from build123d import *

# Parameters (mm, degrees)
BOSS_EXTRUDE1_DEPTH     = 20.95
BOSS_EXTRUDE2_DEPTH     = 9.05
SKETCH6_R               = 2
CUT_EXTRUDE2_DEPTH      = 10
CUT_EXTRUDE3_DEPTH      = 2.75
SKETCH8_W               = 8.290514233
SKETCH8_H               = 3.25
CUT_EXTRUDE4_DEPTH      = 1
CUT_EXTRUDE4_DEPTH_BACK = 31
SKETCH11_R              = 11.15
BEARING_HOLE_DEPTH      = 7.3
SKETCH9_W               = 12.1
SKETCH9_H               = 21.5
WIRE_HOLE_DEPTH         = 15.75
SKETCH12_W              = 46
SKETCH12_H              = 30
BOSS_EXTRUDE3_DEPTH     = 0.0001
BOSS_EXTRUDE4_DEPTH     = 7.5
BOSS_EXTRUDE5_DEPTH     = 7.5
BOSS_EXTRUDE9_DEPTH     = 2.5
SKETCH15_R              = 4
CUT_EXTRUDE5_DEPTH      = 49.5
SKETCH17_R              = 6.169612062
BOSS_EXTRUDE6_DEPTH     = 10
SKETCH18_R              = 3.85
BOSS_EXTRUDE7_DEPTH     = 14
SKETCH19_R              = 4.675
CUT_EXTRUDE6_DEPTH      = 2
SKETCH24_R              = 3.5
CUT_EXTRUDE7_DEPTH      = 23.7
FILLET1_R               = 0.5
SKETCH25_W              = 8.843315878
SKETCH25_H              = 4.834346013
BOSS_EXTRUDE10_DEPTH    = 2
SKETCH27_W              = 12.1
SKETCH27_H              = 21.5
CUT_EXTRUDE8_DEPTH      = 50.7501
BOSS_EXTRUDE11_DEPTH    = 14.7501
SKETCH29_W              = 15.1
SKETCH29_H              = 3
CUT_EXTRUDE9_DEPTH      = 20.95
SKETCH30_R              = 4
CUT_EXTRUDE10_DEPTH     = 14
CUT_EXTRUDE11_DEPTH     = 3


with BuildPart() as part:
    # Sketch2 → Boss-Extrude1 (new body)
    with BuildSketch(Plane.XY):
        with BuildLine():
            Line((-14.709485767, 40), (-23, 40))
            Line((-23, 40), (-23, 0))
            Line((-23, 0), (23, 0))
            Line((23, 0), (23, 40))
            Line((23, 40), (14.709485767, 40))
            ThreePointArc((14.709485767, 40), (0, 54.709485767), (-14.709485767, 40))
        make_face()
        with BuildLine():
            Line((-7.55, 18.241114036), (-7.55, 14.75))
            Line((-7.55, 14.75), (7.55, 14.75))
            Line((7.55, 14.75), (7.55, 18.241114036))
            Line((7.55, 18.241114036), (9.25, 18.241114036))
            Line((9.25, 18.241114036), (9.25, 21.160258306))
            ThreePointArc((9.25, 21.160258306), (0, 46.25), (-9.25, 21.160258306))
            Line((-9.25, 21.160258306), (-9.25, 18.241114036))
            Line((-9.25, 18.241114036), (-7.55, 18.241114036))
        make_face(mode=Mode.SUBTRACT)
    extrude(amount=BOSS_EXTRUDE1_DEPTH)

    # Sketch3 → Boss-Extrude2 (add)
    with BuildSketch(Plane.XY):
        with BuildLine():
            Line((-14.709485767, 40), (-23, 40))
            Line((-23, 40), (-23, 0))
            Line((-23, 0), (23, 0))
            Line((23, 0), (23, 40))
            Line((23, 40), (14.709485767, 40))
            ThreePointArc((14.709485767, 40), (0, 54.709485767), (-14.709485767, 40))
        make_face()
    extrude(amount=-BOSS_EXTRUDE2_DEPTH)

    # Sketch6 → Cut-Extrude2 (cut)
    with BuildSketch(Plane.XY.offset(20.95)):
        with Locations((-17.5, 32)):
            Circle(SKETCH6_R)
        with Locations((17.5, 32)):
            Circle(SKETCH6_R)
    extrude(amount=-CUT_EXTRUDE2_DEPTH, mode=Mode.SUBTRACT)

    # Sketch7 → Cut-Extrude3 (cut)
    with BuildSketch(Plane.XY.offset(20.95)):
        with BuildLine():
            Line((-17.5, 35.75), (17.5, 35.75))
            ThreePointArc((17.5, 35.75), (21.25, 32), (17.5, 28.25))
            Line((17.5, 28.25), (-17.5, 28.25))
            ThreePointArc((-17.5, 28.25), (-21.25, 32), (-17.5, 35.75))
        make_face()
    extrude(amount=-CUT_EXTRUDE3_DEPTH, mode=Mode.SUBTRACT)

    # Sketch8 → Cut-Extrude4 (cut, two sides)
    with BuildSketch(Plane.XY.offset(20.95)) as cut_extrude4_sk:
        with Locations((-18.854742884, 38.375)):
            Rectangle(SKETCH8_W, SKETCH8_H)
        with Locations((18.854742884, 38.375)):
            Rectangle(SKETCH8_W, SKETCH8_H)
    extrude(amount=CUT_EXTRUDE4_DEPTH, mode=Mode.SUBTRACT)
    extrude(cut_extrude4_sk.sketch, amount=-CUT_EXTRUDE4_DEPTH_BACK, mode=Mode.SUBTRACT)

    # Sketch11 → Bearing Hole (cut)
    with BuildSketch(Plane(origin=(0, 0, -9.05), x_dir=(-1, 0, 0), z_dir=(0, 0, -1))):
        with Locations((0, 40)):
            Circle(SKETCH11_R)
    extrude(amount=-BEARING_HOLE_DEPTH, mode=Mode.SUBTRACT)

    # Sketch9 → Wire Hole (cut, through all)
    with BuildSketch(Plane(origin=(0, 14.75, -19.25), x_dir=(-1, 0, 0), z_dir=(0, 1, 0))):
        with Locations((0, 26.95)):
            Rectangle(SKETCH9_W, SKETCH9_H)
    extrude(amount=-WIRE_HOLE_DEPTH, mode=Mode.SUBTRACT)

    # Sketch12 → Boss-Extrude3 (add)
    with BuildSketch(Plane.XZ):
        with Locations((0, 5.95)):
            Rectangle(SKETCH12_W, SKETCH12_H)
    extrude(amount=BOSS_EXTRUDE3_DEPTH)

    # Sketch13 → Boss-Extrude4 (add)
    with BuildSketch(Plane(origin=(23, 0, 0), x_dir=(0, 0, -1), z_dir=(1, 0, 0))):
        with BuildLine():
            Line((-20.95, -0.0001), (-20.95, -20.0001))
            ThreePointArc((-20.95, -20.0001), (-5.95, -35.0001), (9.05, -20.0001))
            Line((9.05, -20.0001), (9.05, -0.0001))
            Line((9.05, -0.0001), (-20.95, -0.0001))
        make_face()
    extrude(amount=-BOSS_EXTRUDE4_DEPTH)

    # Sketch14 → Boss-Extrude5 (add)
    with BuildSketch(Plane.ZY.offset(23)):
        with BuildLine():
            Line((-9.05, -20.0001), (-9.05, -0.0001))
            Line((-9.05, -0.0001), (20.95, -0.0001))
            Line((20.95, -0.0001), (20.95, -20.0001))
            ThreePointArc((20.95, -20.0001), (5.95, -35.0001), (-9.05, -20.0001))
        make_face()
    extrude(amount=-BOSS_EXTRUDE5_DEPTH)

    # Sketch21 → Boss-Extrude9 (add)
    with BuildSketch(Plane(origin=(23, 0, 0), x_dir=(0, 0, -1), z_dir=(1, 0, 0))):
        with BuildLine():
            Line((-20.95, -20.0001), (-20.95, 36.75))
            Line((-20.95, 36.75), (9.05, 36.75))
            Line((9.05, 36.75), (9.05, -20.0001))
            ThreePointArc((9.05, -20.0001), (-5.95, -35.0001), (-20.95, -20.0001))
        make_face()
    extrude(amount=BOSS_EXTRUDE9_DEPTH)

    # Sketch15 → Cut-Extrude5 (cut, through all)
    with BuildSketch(Plane.ZY.offset(23)):
        with Locations((5.95, -20.0001)):
            Circle(SKETCH15_R)
    extrude(amount=-CUT_EXTRUDE5_DEPTH, mode=Mode.SUBTRACT)

    # Sketch17 → Boss-Extrude6 (add)
    with BuildSketch(Plane(origin=(25.5, 0, -23), x_dir=(0, 0, 1), z_dir=(-1, 0, 0))):
        with Locations((28.95, -20.0001)):
            Circle(SKETCH17_R)
        with BuildLine():
            Line((26.765394773, -18.5001), (31.134605227, -18.5001))
            ThreePointArc((31.134605227, -18.5001), (31.6, -20.0001), (31.134605227, -21.5001))
            Line((31.134605227, -21.5001), (26.765394773, -21.5001))
            ThreePointArc((26.765394773, -21.5001), (26.3, -20.0001), (26.765394773, -18.5001))
        make_face(mode=Mode.SUBTRACT)
    extrude(amount=BOSS_EXTRUDE6_DEPTH)

    # Sketch19 → Cut-Extrude6 (cut)
    with BuildSketch(Plane.ZY.offset(-15.5)):
        with Locations((5.95, -20.0001)):
            Circle(SKETCH19_R)
    extrude(amount=-CUT_EXTRUDE6_DEPTH, mode=Mode.SUBTRACT)

    # Sketch24 → Cut-Extrude7 (cut, through all)
    with BuildSketch(Plane(origin=(0, 0, -1.75), x_dir=(-1, 0, 0), z_dir=(0, 0, -1))):
        with Locations((0, 40)):
            Circle(SKETCH24_R)
    extrude(amount=-CUT_EXTRUDE7_DEPTH, mode=Mode.SUBTRACT)

    # Fillet1
    fillet1_edges = [part.edges().sort_by_distance(p)[0] for p in [
        (11.15, 40, -9.05),
    ]]
    fillet(fillet1_edges, radius=FILLET1_R)

    # Sketch25 → Boss-Extrude10 (add)
    with BuildSketch(Plane(origin=(25.5, 0, 0), x_dir=(0, 0, -1), z_dir=(1, 0, 0))):
        with Locations((-6.185865257, -20.38943492)):
            Rectangle(SKETCH25_W, SKETCH25_H)
    extrude(amount=-BOSS_EXTRUDE10_DEPTH)

    # Sketch27 → Cut-Extrude8 (cut, through all)
    with BuildSketch(Plane(origin=(0, 14.75, 0), x_dir=(1, 0, 0), z_dir=(0, 1, 0))):
        with Locations((0, -7.7)):
            Rectangle(SKETCH27_W, SKETCH27_H)
    extrude(amount=-CUT_EXTRUDE8_DEPTH, mode=Mode.SUBTRACT)

    # Sketch28 → Boss-Extrude11 (add)
    with BuildSketch(Plane.XZ.offset(0.0001)):
        Polygon((-6.05, 7.7), (0, 17.95), (6.05, 7.7), (6.05, 18.45), (-6.05, 18.45), align=None)
    extrude(amount=-BOSS_EXTRUDE11_DEPTH)

    # Sketch29 → Cut-Extrude9 (cut)
    with BuildSketch(Plane.XY.offset(20.95)):
        with Locations((0, 13.25)):
            Rectangle(SKETCH29_W, SKETCH29_H)
    extrude(amount=-CUT_EXTRUDE9_DEPTH, mode=Mode.SUBTRACT)

    # Sketch31 → Cut-Extrude11 (cut)
    with BuildSketch(Plane.ZY.offset(23)):
        Polygon((5.95, -10.0001), (15.95, -20.0001), (5.95, -30.0001), (-4.05, -20.0001), align=None)
    extrude(amount=-CUT_EXTRUDE11_DEPTH, mode=Mode.SUBTRACT)


with BuildPart() as body_2:
    # Sketch18 → Boss-Extrude7 (new body)
    with BuildSketch(Plane.ZY.offset(23)):
        with Locations((5.95, -20.0001)):
            Circle(SKETCH18_R)
    extrude(amount=-BOSS_EXTRUDE7_DEPTH)

    # Sketch30 → Cut-Extrude10 (cut)
    with BuildSketch(Plane.ZY.offset(23)):
        with Locations((5.95, -20.0001)):
            Circle(SKETCH30_R)
    extrude(amount=-CUT_EXTRUDE10_DEPTH, mode=Mode.SUBTRACT)


solid = part.part
Geometry check sheet. Reference: the model listing, model coordinates, mm. A direction names the side the tool comes from. Coordinates: 2 decimals unless noted, no trailing zeros. Loops run counter-clockwise (first coordinate to the right, second up) from the corner with the lowest first, then second, coordinate; pieces in that order, holes last. Notation, with made-up numbers: (61.25, 82.5) - (105.25, 82.5) arc R34 cw to (105.25, 120.5) - close; hole circle Ø3 at (11.25, -11). An arc over 180 degrees is marked (long way). Use one line per item in the form item = value. Start each with the question number.
Item 1: Section check A-A, the plane y = 8.5. Enter the section's corners in (x, z), and give its area (3 significant figures).
Item 2: Section check B-B, the plane z = -5. Enter the section's corners in (x, y), and give its area (3 significant figures).
Item 3: Tool access check on faces 1 (the face through (2.98, 5.79, 12.9)), 2 (the face through (16, 30, 18.2)), 3 (the face through (-21.52, -14.93, 10.88)), 4 (the face through (17.5, -22, 6)). Record the directions out of +Z, -Z, +X, -X, +Y, -Y that give a thin tool (end or side, any length) a straight path to the whole face; none if there is none.
Item 4: Mould release check, pull along Z, two halves, no side actions. Record for faces 5 (the face through (-16, 30, 18.2)), 6 (the face through (20, 36.75, 6)), 7 (the face through (21, -18.5, 6)): +Z half, -Z half, draft (parallel to the pull), parting line (faces both ways), or undercut.
Item 5: Gauge pin test, flat ends, axial feed: pin 1 (3.5 mm diameter, centred on x = 20.5, z = 5, fed in from +Y); pin 2 (1 mm diameter, centred on x = -4.5, z = 16.5, fed in from -Y); pin 3 (1.4 mm diameter, centred on x = 8.5, z = 11.5, fed in from +Y). Record the tip position at first contact, or that the pin passes through.
Item 6: Section check C-C, the plane y = -28.5. Enter the section's corners in (x, z).
Item 7: Thickness scan on probe 1 along X at (y, z) = (-19.5, 19.5); probe 2 along Y at (x, z) = (-17.95, 5.95); probe 3 along X at (y, z) = (13, 17). Record the ranges inside material, lowest first.
Item 8: Section check D-D, the plane x = -2. Give the number of separate pieces and of enclosed holes in the cut face, and give its area (3 significant figures).
Computed:
q1.outline = (-23, -9.05) - (25.5, -9.05) - (25.5, 20.95) - (-23, 20.95) - close; hole (-6.05, -3.05) - (6.05, -3.05) - (6.05, 7.7) - (0, 17.95) - (-6.05, 7.7) - close
q1.area = 1,260 mm2
q2.outline = (-23, -30.25) - (-15.5, -30.25) - (-15.5, 0) - (15.5, 0) - (15.5, -30.25) - (25.5, -30.25) - (25.5, 36.75) - (14.71, 36.75) - (14.71, 40) arc R14.71 ccw to (-14.71, 40) - (-14.71, 36.75) - (-23, 36.75) - close; hole circle Ø22.3 at (0, 40)
q2.area = 2,360 mm2
q3.face_1 = -Y
q3.face_2 = +Z
q3.face_3 = -X
q3.face_4 = none
q4.face_5 = +Z half
q4.face_6 = draft
q4.face_7 = undercut
q5.pin_1 = 36.75
q5.pin_2 = 0
q5.pin_3 = 52.47
q6.outline = (-23, -6.41) - (-15.5, -6.41) - (-15.5, 18.31) - (-23, 18.31) - (-23, 7.45) - (-20, 7.45) - (-20, 4.45) - (-23, 4.45) - close; (15.5, -6.41) - (25.5, -6.41) - (25.5, 18.31) - (15.5, 18.31) - close
q7.probe_1 = -23 to -15.5, 15.5 to 25.5
q7.probe_2 = -35 to -24, -16 to 36.75
q7.probe_3 = -23 to -7.55, 7.55 to 25.5
q8.separate_pieces = 3
q8.enclosed_holes = 0
q8.area = 531 mm2
